Check sheet for the modelled part. Datum: model origin and axes. Units: mm. Face numbers are marked on the shaded views. A direction names the side the tool comes from. Round coordinates to 2 decimals unless told otherwise and drop trailing zeros. Order: outer loops, then holes, each group sorted by start corner. A loop starts at its lowest first (then second) coordinate and runs counter-clockwise, first axis right, second up.
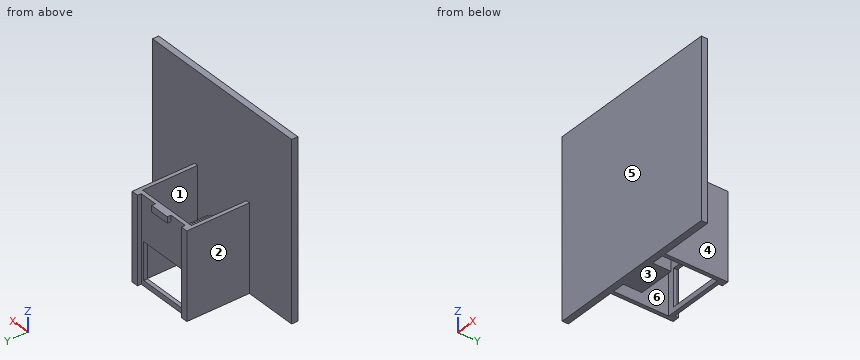
```python
from build123d import *

# Parameters (mm, degrees)
BOSS_EXTRUDE2_DEPTH  = 28
SKETCH4_W            = 6.4
SKETCH4_H            = 26
CUT_EXTRUDE2_DEPTH   = 1.2
SKETCH5_W            = 16
SKETCH5_H            = 12
CUT_EXTRUDE3_DEPTH   = 1.2
SKETCH6_W            = 8.8
SKETCH6_H            = 17.8
BOSS_EXTRUDE3_DEPTH  = 2
SKETCH7_W            = 12
SKETCH7_H            = 6
BOSS_EXTRUDE4_DEPTH  = 15.7
SKETCH8_W            = 1.6
SKETCH8_H            = 6
CUT_EXTRUDE4_DEPTH   = 1
BOSS_EXTRUDE10_DEPTH = 57


with BuildPart() as part:
    # Sketch1 → Boss-Extrude2 (new body)
    with BuildSketch(Plane.XY):
        Polygon((9, -3.6), (9, -21.4), (10.2, -21.4), (10.2, -1.2), (8, -1.2), (8, -2.4), (2.2, -2.4), (2.2, -1.2), (-4.2, -1.2), (-4.2, -2.4), (-10, -2.4), (-10, -1.2), (-12.2, -1.2), (-12.2, -21.4), (-11, -21.4), (-11, -3.6), align=None)
    extrude(amount=BOSS_EXTRUDE2_DEPTH)

    # Sketch4 → Cut-Extrude2 (cut)
    with BuildSketch(Plane(origin=(0, -1.2, 0), x_dir=(1, 0, 0), z_dir=(0, 1, 0))):
        with Locations((-1, -13)):
            Rectangle(SKETCH4_W, SKETCH4_H)
    extrude(amount=-CUT_EXTRUDE2_DEPTH, mode=Mode.SUBTRACT)

    # Sketch5 → Cut-Extrude3 (cut)
    with BuildSketch(Plane(origin=(0, -2.4, 0), x_dir=(1, 0, 0), z_dir=(0, 1, 0))):
        with Locations((-1, -7.7)):
            Rectangle(SKETCH5_W, SKETCH5_H)
    extrude(amount=-CUT_EXTRUDE3_DEPTH, mode=Mode.SUBTRACT)

    # Sketch6 → Boss-Extrude3 (add)
    with BuildSketch(Plane(origin=(0, 0, 13.7), x_dir=(-1, 0, 0), z_dir=(0, 0, -1))):
        with Locations((1, -12.5)):
            Rectangle(SKETCH6_W, SKETCH6_H)
    extrude(amount=-BOSS_EXTRUDE3_DEPTH)

    # Sketch7 → Boss-Extrude4 (add)
    with BuildSketch(Plane.XY.offset(15.7)):
        with Locations((-1, -18.4)):
            Rectangle(SKETCH7_W, SKETCH7_H)
    extrude(amount=-BOSS_EXTRUDE4_DEPTH)

    # Sketch8 → Cut-Extrude4 (cut)
    with BuildSketch(Plane.XY.offset(15.7)):
        with Locations((-6.2, -18.4)):
            Rectangle(SKETCH8_W, SKETCH8_H)
        with Locations((4.2, -18.4)):
            Rectangle(SKETCH8_W, SKETCH8_H)
    extrude(amount=-CUT_EXTRUDE4_DEPTH, mode=Mode.SUBTRACT)

    # Sketch9 → Boss-Extrude10 (add)
    with BuildSketch(Plane(origin=(0, 0, 0), x_dir=(-1, 0, 0), z_dir=(0, 0, -1))):
        Polygon((1, -21.4), (29.5, -21.4), (29.5, -23.4), (-27.5, -23.4), (-27.5, -21.4), align=None)
    extrude(amount=-BOSS_EXTRUDE10_DEPTH)


solid = part.part
```
Item 1: Sectioned sample at C-C (z = 51). Record the cut outline in (x, y).
Answer:
outline: (-29.5, -23.4) - (27.5, -23.4) - (27.5, -21.4) - (-29.5, -21.4) - close
Item 2: Sectioned sample at A-A (x = -2.5). Record the cut outline in (y, z), and give its area (3 significant figures).
Answer:
outline: (-23.4, 0) - (-15.4, 0) - (-15.4, 13.7) - (-2.4, 13.7) - (-2.4, 26) - (-1.2, 26) - (-1.2, 28) - (-3.6, 28) - (-3.6, 15.7) - (-21.4, 15.7) - (-21.4, 57) - (-23.4, 57) - close; (-3.6, 0) - (-2.4, 0) - (-2.4, 1.7) - (-3.6, 1.7) - close
area: 253 mm2
Item 3: Access from +Z, -Z, +X, -X, +Y, -Y to the whole of each face (thin tool, end or side, straight path). Record for the marked faces 5 and 6.
Answer:
face 5: +Z, -Z, +X, -X, -Y
face 6: +Z, -Z
Item 4: Scan lines: line 1 along X through (y, z) = (-3.75, 15); line 2 along X through (y, z) = (-21.25, 7.5); line 3 along X through (y, z) = (-16.25, 25). Record each from-to range of solid material in increasing order.
Answer:
line 1: x = -12.2 to -11, -5.4 to 3.4, 9 to 10.2
line 2: x = -12.2 to -11, -7 to 5, 9 to 10.2
line 3: x = -12.2 to -11, 9 to 10.2
Item 5: Go/stop test with flat-tipped pins: P1, Ø1, axis at y = -15, z = 15, coming from the +X side; P2, Ø1, axis at y = -1.5, z = 17.5, coming from the -X side; P3, Ø4, axis at x = 9, y = -19.5, coming from the -Z side; P4, Ø1.5, axis at x = 11.5, y = -9.5, coming from the +Z side. Record where each tip stops, or that it passes through.
Answer:
P1: stops at x = 10.2
P2: stops at x = -12.2
P3: stops at z = 0
P4: passes through
Item 6: Sectioned sample at B-B (y = -19.75). Record the cut outline in (x, z).
Answer:
outline: (-12.2, 0) - (-11, 0) - (-11, 28) - (-12.2, 28) - close; (-7, 0) - (5, 0) - (5, 14.7) - (3.4, 14.7) - (3.4, 15.7) - (-5.4, 15.7) - (-5.4, 14.7) - (-7, 14.7) - close; (9, 0) - (10.2, 0) - (10.2, 28) - (9, 28) - close
Item 7: Sectioned sample at D-D (y = -14.5). Record the cut outline in (x, z), and give its area (3 significant figures).
Answer:
outline: (-12.2, 0) - (-11, 0) - (-11, 28) - (-12.2, 28) - close; (-5.4, 13.7) - (3.4, 13.7) - (3.4, 15.7) - (-5.4, 15.7) - close; (9, 0) - (10.2, 0) - (10.2, 28) - (9, 28) - close
area: 84.8 mm2
Item 8: Release check for a two-part mould opening along X. For the marked faces 1, 2, 3 and 4 record: released by +X, released by -X, zero draft, split by the parting line, or undercut.
Answer:
face 1: undercut
face 2: released by -X
face 3: zero draft
face 4: released by +X
